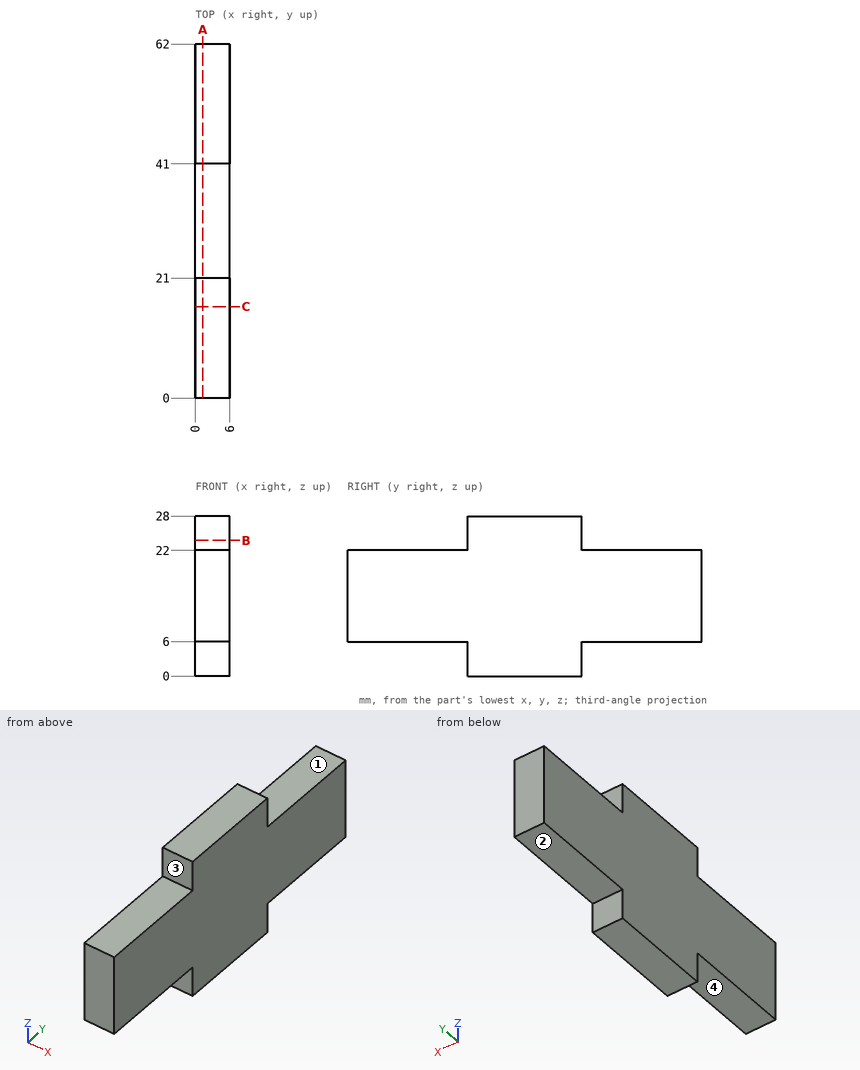
Verification items for this drawing (mm, ordinates from the low corner). A direction names the side the tool comes from. Coordinates: 2 decimals unless noted, no trailing zeros. Write each loop counter-clockwise with the first axis right and the second up, starting at its lowest first coordinate (ties: lowest second). Pieces come first, ordered by that corner, then holes. Notation, with made-up numbers: M -15,-21.5 L 25,-21.5 A20 cw 25,3.5 Z; hole C 47.25,67.25 d3. An arc over 180 degrees is marked long. Answer as a JSON object with one key per item and string values. Group by question number.
(1) Gauge pin test, flat ends, axial feed: pin 1 (2 mm diameter, centred on x = 5, z = 3, fed in from -Y); pin 2 (1.8 mm diameter, centred on x = 2.5, z = 23.5, fed in from +Y); pin 3 (1.8 mm diameter, centred on x = 2.5, y = 15, fed in from -Z). Record the tip position at first contact, or that the pin passes through.
(2) Cross-section at A-A, the plane x = 1.3. Record the cut outline in (y, z), and give its area (3 significant figures).
(3) Tool access check on the marked faces 1, 2, 3 and 4. Record the directions out of +Z, -Z, +X, -X, +Y, -Y that give a thin tool (end or side, any length) a straight path to the whole face; none if there is none.
(4) Material ranges on line 1 (Z direction, x = 4.7, y = 5.5); line 2 (Y direction, x = 0.45, z = 4), recorded low to high.
(5) Cross-section at C-C, the plane y = 16. Record the cut outline in (x, z).
(6) Cross-section at B-B, the plane z = 23.75. Record the cut outline in (x, y).
Reply:
{
 "1": {"pin 1": "y = 21", "pin 2": "y = 41", "pin 3": "z = 6"},
 "2": {"outline": "M 0,6 L 21,6 L 21,0 L 41,0 L 41,6 L 62,6 L 62,22 L 41,22 L 41,28 L 21,28 L 21,22 L 0,22 Z", "area": "1,230 mm²"},
 "3": {"face 1": "+Z, +X, -X, +Y", "face 2": "-Z, +X, -X, +Y", "face 3": "+Z, +X, -X, -Y", "face 4": "-Z, +X, -X, -Y"},
 "4": {"line 1": "6 to 22", "line 2": "21 to 41"},
 "5": {"outline": "M 0,6 L 6,6 L 6,22 L 0,22 Z"},
 "6": {"outline": "M 0,21 L 6,21 L 6,41 L 0,41 Z"}
}
